```python
from build123d import *

# Parameters (mm, degrees)
BOSS_EXTRUDE1_DEPTH = 22.86
SKETCH2_R           = 1.5875
BOSS_EXTRUDE2_DEPTH = 2.54
SKETCH4_W           = 15.367
SKETCH4_H           = 22.86
SKETCH4_R           = 3.2639
BOSS_EXTRUDE3_DEPTH = 5.08
SKETCH5_W           = 13.081
SKETCH5_H           = 4.233333333
SKETCH5_H_2         = 4.233333334
BOSS_EXTRUDE4_DEPTH = 12.7
CHAMFER1_SIZE       = 12.7
FILLET1_R           = 2.38


with BuildPart() as part:
    # Sketch1 → Boss-Extrude1 (new body)
    with BuildSketch(Plane.XY):
        Polygon((-3.81, 35.052), (0, 35.052), (0, 0), (72.898, 0), (72.898, 35.052), (76.708, 35.052), (76.708, -3.81), (-3.81, -3.81), align=None)
    extrude(amount=BOSS_EXTRUDE1_DEPTH)

    # Sketch2 → Boss-Extrude2 (add)
    with BuildSketch(Plane.XZ.offset(3.81)):
        with BuildLine():
            ThreePointArc((89.789, 26.6192), (84.709, 31.6992), (79.629, 26.6192))
            Line((79.629, 26.6192), (79.629, 22.86))
            Line((79.629, 22.86), (76.708, 22.86))
            Line((76.708, 22.86), (76.708, 0))
            Line((76.708, 0), (79.629, 0))
            Line((79.629, 0), (79.629, -21.5392))
            ThreePointArc((79.629, -21.5392), (84.709, -26.6192), (89.789, -21.5392))
            Line((89.789, -21.5392), (89.789, 26.6192))
        make_face()
        with Locations((84.709, -21.5392)):
            Circle(SKETCH2_R, mode=Mode.SUBTRACT)
        with Locations((84.709, 26.6192)):
            Circle(SKETCH2_R, mode=Mode.SUBTRACT)
    extrude(amount=-BOSS_EXTRUDE2_DEPTH)

    # Sketch4 → Boss-Extrude3 (add)
    with BuildSketch(Plane(origin=(0, 35.052, 0), x_dir=(1, 0, 0), z_dir=(0, 1, 0))):
        with Locations((-7.6835, -11.43)):
            Rectangle(SKETCH4_W, SKETCH4_H)
        with Locations(Location((-9.525, -3.81, 0), (0, 0, 270))):
            Circle(SKETCH4_R, mode=Mode.SUBTRACT)
        with Locations(Location((-9.525, -19.05, 0), (0, 0, 270))):
            Circle(SKETCH4_R, mode=Mode.SUBTRACT)
    boss_extrude3 = extrude(amount=-BOSS_EXTRUDE3_DEPTH)

    # Mirror1: Boss-Extrude3 across plane
    add(boss_extrude3.mirror(Plane(origin=(36.449, 0, 0), x_dir=(0, 0, 1), z_dir=(1, 0, 0))))

    # Sketch5 → Boss-Extrude4 (add)
    with BuildSketch(Plane(origin=(0, -1.27, 0), x_dir=(1, 0, 0), z_dir=(0, 1, 0))):
        with Locations((83.2485, -2.116666667)):
            Rectangle(SKETCH5_W, SKETCH5_H)
        with Locations((83.2485, -20.743333334)):
            Rectangle(SKETCH5_W, SKETCH5_H)
        with Locations((83.2485, -11.43)):
            Rectangle(SKETCH5_W, SKETCH5_H_2)
    extrude(amount=BOSS_EXTRUDE4_DEPTH)

    # Chamfer1
    chamfer1_edges = [part.edges().sort_by_distance(p)[0] for p in [
        (89.789, 11.43, 20.743333333),
        (89.789, 11.43, 11.43),
        (89.789, 11.43, 2.116666667),
    ]]
    chamfer(chamfer1_edges, length=CHAMFER1_SIZE)

    # Fillet1
    fillet1_edges = [part.edges().sort_by_distance(p)[0] for p in [
        (-3.81, 29.972, 11.43),
        (76.708, 29.972, 11.43),
    ]]
    fillet(fillet1_edges, radius=FILLET1_R)


solid = part.part
```
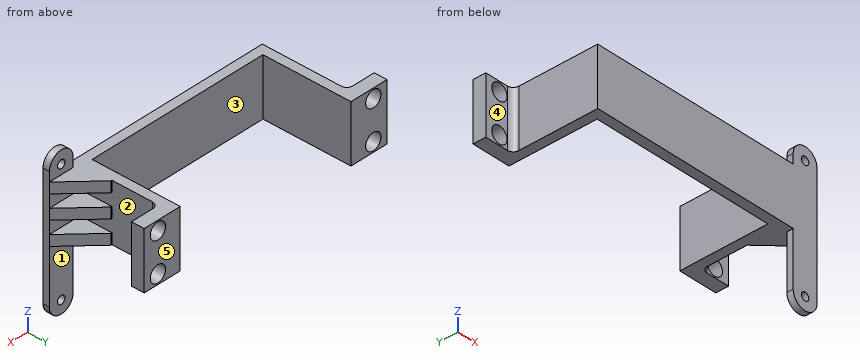
Can you work these out from the model? Positions are in its coordinate system, mm. Face numbers are marked on the shaded views. A direction names the side the tool comes from. Coordinates: 2 decimals unless noted, no trailing zeros. Loops run counter-clockwise (first coordinate to the right, second up) from the corner with the lowest first, then second, coordinate; pieces in that order, holes last. Notation, with made-up numbers: (-18.5, 58) -> (37.5, 58) arc R28 ccw to (37.5, 91) -> close; hole circle Ø11 at (-1.5, 10.25). An arc over 180 degrees is marked (long way). Answer as a JSON object with one key per item and string values.
1) Thinking about a two-plate mould opening in Z: for the marked faces 1 and 2, which applies, pulls with the +Z half, pulls with the -Z half, needs draft (parallel to the pull), parting line crosses it, or undercut?
Results:
{"face 1": "needs draft", "face 2": "undercut"}
2) Imagine slicing it at B-B (x = -8.5). Please give me the cut outline in (y, z), then the cut area to 3 significant figures.
Results:
{"outline": "(29.97, 0) -> (35.05, 0) -> (35.05, 0.71) -> (29.97, 0.71) -> close; (29.97, 6.91) -> (35.05, 6.91) -> (35.05, 15.95) -> (29.97, 15.95) -> close; (29.97, 22.15) -> (35.05, 22.15) -> (35.05, 22.86) -> (29.97, 22.86) -> close", "area": "53.2 mm^2"}
3) For the marked faces 3, 4 and 5, which set-ups out of +Z, -Z, +X, -X, +Y, -Y let a thin tool reach every point of the face, with its end or its side?
Results:
{"face 3": "+Z, -Z, +Y", "face 4": "+Z, -Z, -X, -Y", "face 5": "+Z, -Z, +X, -X, +Y"}
4) Imagine slicing it at A-A (y = 20). Please give me the cut outline in (x, z), then the cut area to 3 significant figures.
Results:
{"outline": "(-3.81, 0) -> (0, 0) -> (0, 22.86) -> (-3.81, 22.86) -> close; (72.9, 0) -> (76.71, 0) -> (76.71, 22.86) -> (72.9, 22.86) -> close", "area": "174 mm^2"}
5) Imagine slicing it at C-C (z = -6). Please give me the cut outline in (x, y).
Results:
{"outline": "(79.63, -3.81) -> (89.79, -3.81) -> (89.79, -1.27) -> (79.63, -1.27) -> close"}
6) Imagine slicing it at D-D (x = 35.5). Please give me the cut outline in (y, z).
Results:
{"outline": "(-3.81, 0) -> (0, 0) -> (0, 22.86) -> (-3.81, 22.86) -> close"}
7) For P1, Ø10, axis at x = 84, y = 3, coming from the -Z side; P2, Ø10, axis at x = 86, y = 8, coming from the -Z side; P3, Ø5, axis at x = 85, z = -19, coming from the +Y side; P4, Ø10, axis at y = 23.5, z = 9, coming from the -X side, each with a flat end and sliding along its axis, tell me the tip position at first contact or that it passes through.
Results:
{"P1": "stops at z = -26.62", "P2": "stops at z = 0", "P3": "stops at y = -1.27", "P4": "stops at x = -3.99"}
8) If I drill on line 1 (X direction, y = 32, z = 19) (3 decimals); line 2 (Y direction, x = 52.5, z = 8.5); line 3 (X direction, y = 12, z = 4), over which ranges is the centre line in solid material (lowest first)?
Results:
{"line 1": "x = -15.367 to -12.789, -6.261 to 0, 72.898 to 79.159, 85.687 to 88.265", "line 2": "y = -3.81 to 0", "line 3": "x = -3.81 to 0, 72.9 to 76.71"}
